Read the model definition and answer for the solid it produces. Units are mm, in the model's axes. Face numbers are marked on the shaded views. A direction names the side the tool comes from. Coordinates: 2 decimals unless noted, no trailing zeros. Write each loop counter-clockwise with the first axis right and the second up, starting at its lowest first coordinate (ties: lowest second). Pieces come first, ordered by that corner, then holes.
(1) Which of the six approach directions +Z, -Z, +X, -X, +Y, -Y give full straight-line access (tool end or side, diameter ignored) to the marked faces 4 and 5?
(2) Section D-D on x = 10 is taken. Write down the section's boundary in (y, z), then the cut area to 3 significant figures.
(3) Section B-B on y = 5 is taken. Write down the section's boundary in (x, z), then the cut area to 3 significant figures.
(4) Find the intervals of material crossed by probe 1 along X at (y, z) = (18.5, 12.5); probe 2 along Z at (x, y) = (-18.5, 26); probe 3 along X at (y, z) = (26, -3), in increasing order.
(5) Section A-A on y = 41.5 is taken. Write down the section's boundary in (x, z), then the cut area to 3 significant figures.
(6) Given pin 1 (15 mm diameter, centred on x = -10, z = -2.5, fed in from +Y); pin 2 (2 mm diameter, centred on y = 20, z = 1, fed in from -X); pin 3 (0.6 mm diameter, centred on x = -51, z = 0.5, fed in from +Y), each flat-ended and moving along its own axis, determine where each tip first touches the part or whether it passes through.
(7) The mould has two halves that part along X. Classify the marked faces 1, 2 and 3: +X half, -X half, draft (parallel to the pull), parting line (faces both ways), or undercut.
(8) Section C-C on z = 11 is taken. Write down the section's boundary in (x, y).
from build123d import *

# Parameters (mm, degrees)
SKETCH1_W           = 104
SKETCH1_H           = 54
SKETCH1_W_2         = 100
SKETCH1_H_2         = 50
BOSS_EXTRUDE1_DEPTH = 45
SKETCH2_W           = 104
SKETCH2_H           = 54
BOSS_EXTRUDE2_DEPTH = 2
SKETCH3_W           = 2
SKETCH3_H           = 5
CUT_EXTRUDE1_DEPTH  = 30
SKETCH4_W           = 2
SKETCH4_H           = 26.201240847
BOSS_EXTRUDE3_DEPTH = 40


with BuildPart() as part:
    # Sketch1 → Boss-Extrude1 (new body)
    with BuildSketch(Plane(origin=(0, 0, 0), x_dir=(1, 0, 0), z_dir=(0, 1, 0))):
        Rectangle(SKETCH1_W, SKETCH1_H)
        Rectangle(SKETCH1_W_2, SKETCH1_H_2, mode=Mode.SUBTRACT)
    extrude(amount=BOSS_EXTRUDE1_DEPTH)

    # Sketch2 → Boss-Extrude2 (add)
    with BuildSketch(Plane(origin=(0, 0, 0), x_dir=(1, 0, 0), z_dir=(0, 1, 0))):
        Rectangle(SKETCH2_W, SKETCH2_H)
    extrude(amount=-BOSS_EXTRUDE2_DEPTH)

    # Sketch3 → Cut-Extrude1 (cut)
    with BuildSketch(Plane(origin=(0, 45, 0), x_dir=(1, 0, 0), z_dir=(0, 1, 0))):
        with Locations((51, 0)):
            Rectangle(SKETCH3_W, SKETCH3_H)
        with Locations((-51, 0)):
            Rectangle(SKETCH3_W, SKETCH3_H)
    extrude(amount=-CUT_EXTRUDE1_DEPTH, mode=Mode.SUBTRACT)

    # Sketch4 → Boss-Extrude3 (add)
    with BuildSketch(Plane(origin=(0, 0, 0), x_dir=(1, 0, 0), z_dir=(0, 1, 0))):
        with Locations((21, -11.899379576)):
            Rectangle(SKETCH4_W, SKETCH4_H)
    extrude(amount=BOSS_EXTRUDE3_DEPTH)


solid = part.part
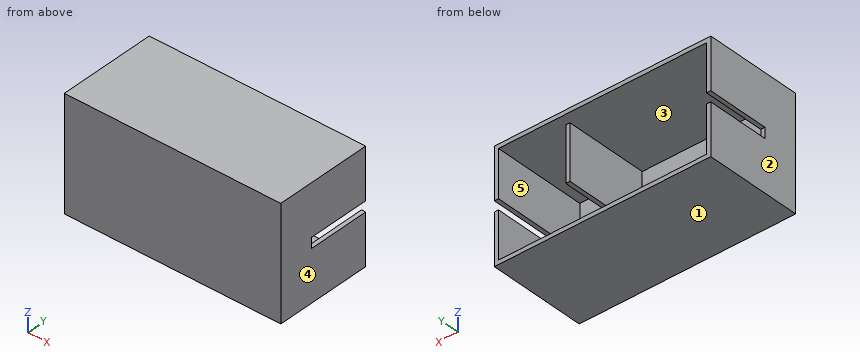
Response:
1. face 4: +Z, -Z, +X, +Y, -Y
1. face 5: +Y
2. outline: (-2, -27) - (45, -27) - (45, -25) - (0, -25) - (0, 25) - (45, 25) - (45, 27) - (-2, 27) - close
2. area: 288 mm2
3. outline: (-52, -27) - (52, -27) - (52, 27) - (-52, 27) - close; hole (-50, -25) - (50, -25) - (50, 25) - (22, 25) - (22, -1.2) - (20, -1.2) - (20, 25) - (-50, 25) - close
3. area: 668 mm2
4. probe 1: x = -52 to -50, 20 to 22, 50 to 52
4. probe 2: z = -27 to -25, 25 to 27
4. probe 3: x = -52 to -50, 50 to 52
5. outline: (-52, -27) - (52, -27) - (52, -2.5) - (50, -2.5) - (50, -25) - (-50, -25) - (-50, -2.5) - (-52, -2.5) - close; (-52, 2.5) - (-50, 2.5) - (-50, 25) - (50, 25) - (50, 2.5) - (52, 2.5) - (52, 27) - (-52, 27) - close
5. area: 596 mm2
6. pin 1: stops at y = 0
6. pin 2: stops at x = 20
6. pin 3: stops at y = 15
7. face 1: draft
7. face 2: -X half
7. face 3: undercut
8. outline: (-52, -2) - (52, -2) - (52, 45) - (50, 45) - (50, 0) - (22, 0) - (22, 40) - (20, 40) - (20, 0) - (-50, 0) - (-50, 45) - (-52, 45) - close
